from build123d import *

# Parameters (mm, degrees)
CROQUIS1_W              = 250
CROQUIS1_H              = 130
SALIENTE_EXTRUIR1_DEPTH = 1.0555
CROQUIS3_W              = 250
CROQUIS3_H              = 90
SALIENTE_EXTRUIR2_DEPTH = 2.11
CROQUIS4_W              = 100
CROQUIS4_H              = 50
CORTAR_EXTRUIR1_DEPTH   = 2.111
CROQUIS5_W              = 134.22
CROQUIS5_H              = 90
SALIENTE_EXTRUIR3_DEPTH = 2.11


with BuildPart() as part:
    # Croquis1 → Saliente-Extruir1 (new body, symmetric)
    with BuildSketch(Plane(origin=(0, 0, 0), x_dir=(1, 0, 0), z_dir=(0, 1, 0))):
        Rectangle(CROQUIS1_W, CROQUIS1_H)
    extrude(amount=SALIENTE_EXTRUIR1_DEPTH, both=True)

    # Croquis3 → Saliente-Extruir2 (add)
    with BuildSketch(Plane.XY.offset(65)):
        with Locations((0, 43.9445)):
            Rectangle(CROQUIS3_W, CROQUIS3_H)
    saliente_extruir2 = extrude(amount=SALIENTE_EXTRUIR2_DEPTH)

    # Simetría1: Saliente-Extruir2 across plane
    add(saliente_extruir2.mirror(Plane.XY))

    # Croquis4 → Cortar-Extruir1 (cut)
    with BuildSketch(Plane(origin=(0, 1.0555, 0), x_dir=(1, 0, 0), z_dir=(0, 1, 0))):
        Rectangle(CROQUIS4_W, CROQUIS4_H)
    extrude(amount=-CORTAR_EXTRUIR1_DEPTH, mode=Mode.SUBTRACT)

    # Croquis5 → Saliente-Extruir3 (add)
    with BuildSketch(Plane.ZY.offset(125)):
        with Locations((0, 43.9445)):
            Rectangle(CROQUIS5_W, CROQUIS5_H)
    extrude(amount=SALIENTE_EXTRUIR3_DEPTH)


solid = part.part
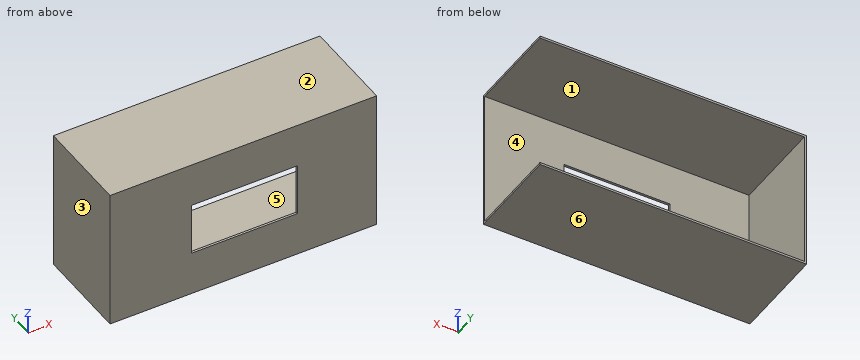
Work out the finished part from the listing and answer in its coordinate system (mm). Face numbers are marked on the shaded views. A direction names the side the tool comes from. Round coordinates to 2 decimals unless told otherwise and drop trailing zeros. Order: outer loops, then holes, each group sorted by start corner. A loop starts at its lowest first (then second) coordinate and runs counter-clockwise, first axis right, second up. Notation, with made-up numbers: M 4.25,52.25 L 53.25,52.25 A19 ccw 53.25,73.25 Z; hole C 34,-23 d5. An arc over 180 degrees is marked long. One line per item, written item: value.
Q1. Find section A-A on z = 21. Write down the section's boundary in (x, y), then the cut area to 3 significant figures.
Derived:
outline: M -127.11,-1.06 L -50,-1.06 L -50,1.06 L -125,1.06 L -125,88.94 L -127.11,88.94 Z; M 50,-1.06 L 125,-1.06 L 125,1.06 L 50,1.06 Z
area: 507 mm²
Q2. Find section C-C on y = 44.5. Write down the section's boundary in (x, z).
Derived:
outline: M -127.11,-67.11 L 125,-67.11 L 125,-65 L -125,-65 L -125,65 L 125,65 L 125,67.11 L -127.11,67.11 Z
Q3. Find section D-D on z = 47. Write down the section's boundary in (x, y).
Derived:
outline: M -127.11,-1.06 L 125,-1.06 L 125,1.06 L -125,1.06 L -125,88.94 L -127.11,88.94 Z
Q4. For the marked faces 5 and 6, determine the directions among +Z, -Z, +X, -X, +Y, -Y from which every point of the face is accessible in a straight line to the end or side of a thin tool.
Derived:
face 5: +X, +Y
face 6: -Z, +X, -X, +Y, -Y
Q5. Flat-ended cylindrical pins translate along their axes: pin 1 (6 mm diameter, centred on x = 83, z = -22, fed in from +Y); pin 2 (5 mm diameter, centred on y = 68.5, z = -1, fed in from +X). Find the tip coordinate at first contact, or state that the pin passes through.
Derived:
pin 1: y = 1.06
pin 2: x = -125
Q6. Straight lines are drawn through the part: line 1 (Z direction, x = -27, y = 85); line 2 (X direction, y = 20.5, z = -52.5); line 3 (Y direction, x = 11.5, z = 44.5). For each, find the intervals that lie inside material, in ascending order.
Derived:
line 1: -67.11 to -65, 65 to 67.11
line 2: -127.11 to -125
line 3: -1.06 to 1.06
Q7. Determine the mould class of the marked faces 1, 2, 3 and 4 for opening direction Z: released by +Z, released by -Z, zero draft, split by the parting line, or undercut.
Derived:
face 1: undercut
face 2: released by +Z
face 3: zero draft
face 4: undercut
Q8. Find section B-B on x = 47.5. Write down the section's boundary in (y, z), then the cut area to 3 significant figures.
Derived:
outline: M -1.06,-67.11 L 88.94,-67.11 L 88.94,-65 L 1.06,-65 L 1.06,-25 L -1.06,-25 Z; M -1.06,25 L 1.06,25 L 1.06,65 L 88.94,65 L 88.94,67.11 L -1.06,67.11 Z
area: 549 mm²
